Here's how the part is built. I have some questions about the finished solid (model axes, mm). Face numbers are marked on the shaded views. Give positions to 0.01 mm unless a question says otherwise; leave off trailing zeros. Loops run counter-clockwise (first coordinate to the right, second up) from the corner with the lowest first, then second, coordinate; pieces in that order, holes last. Notation, with made-up numbers: (-19, -30) - (17, -30) arc R21 cw to (17, -19) - close; hole circle Ø11 at (49.25, 32). An arc over 180 degrees is marked (long way). Use one line per item in the form item = value.
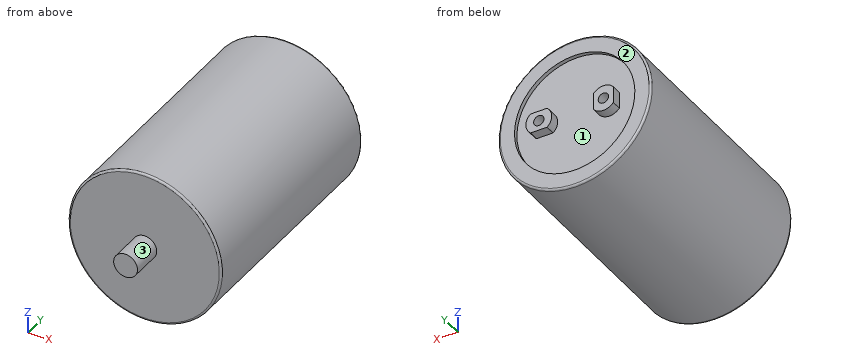
from build123d import *

# Parameters (mm, degrees)
SKETCH1_R           = 38.5
BOSS_EXTRUDE1_DEPTH = 115
SKETCH2_R           = 2.6
BOSS_EXTRUDE2_DEPTH = 5
SKETCH3_R           = 38.5
SKETCH3_R_2         = 30.3
BOSS_EXTRUDE3_DEPTH = 2
FILLET1_R           = 1
ESQUISSE1_R         = 6
BOSS_EXTRU_1_DEPTH  = 16


with BuildPart() as part:
    # Sketch1 → Boss-Extrude1 (new body)
    with BuildSketch(Plane(origin=(0, 0, 0), x_dir=(1, 0, 0), z_dir=(0, 1, 0))):
        with Locations(Location((0, 0, 0), (0, 0, 270))):
            Circle(SKETCH1_R)
    extrude(amount=BOSS_EXTRUDE1_DEPTH)

    # Sketch2 → Boss-Extrude2 (add)
    # profile 1 of 2: a face of its own
    with BuildSketch(Plane(origin=(0, 115, 0), x_dir=(1, 0, 0), z_dir=(0, 1, 0))):
        with BuildLine():
            Line((-21.25, 4.153311931), (-21.25, -4.153311931))
            ThreePointArc((-21.25, -4.153311931), (-16.25, -6.5), (-11.25, -4.153311931))
            Line((-11.25, -4.153311931), (-11.25, 4.153311931))
            ThreePointArc((-11.25, 4.153311931), (-16.25, 6.5), (-21.25, 4.153311931))
        make_face()
        with Locations(Location((-16.25, 0, 0), (0, 0, 270))):
            Circle(SKETCH2_R, mode=Mode.SUBTRACT)
    # profile 2 of 2: a face of its own
    with BuildSketch(Plane(origin=(0, 115, 0), x_dir=(1, 0, 0), z_dir=(0, 1, 0))):
        with BuildLine():
            Line((12.096688069, 5), (20.403311931, 5))
            ThreePointArc((20.403311931, 5), (22.75, 0), (20.403311931, -5))
            Line((20.403311931, -5), (12.096688069, -5))
            ThreePointArc((12.096688069, -5), (9.75, 0), (12.096688069, 5))
        make_face()
        with Locations(Location((16.25, 0, 0), (0, 0, 270))):
            Circle(SKETCH2_R, mode=Mode.SUBTRACT)
    extrude(amount=BOSS_EXTRUDE2_DEPTH)

    # Sketch3 → Boss-Extrude3 (add)
    with BuildSketch(Plane(origin=(0, 115, 0), x_dir=(1, 0, 0), z_dir=(0, 1, 0))):
        with Locations(Location((0, 0, 0), (0, 0, 270))):
            Circle(SKETCH3_R)
        with Locations(Location((0, 0, 0), (0, 0, 270))):
            Circle(SKETCH3_R_2, mode=Mode.SUBTRACT)
    extrude(amount=BOSS_EXTRUDE3_DEPTH)

    # Fillet1
    fillet1_edges = [part.edges().sort_by_distance(p)[0] for p in [
        (0, 0, -38.5),
        (0, 117, -38.5),
    ]]
    fillet(fillet1_edges, radius=FILLET1_R)

    # Esquisse1 → Boss.-Extru.1 (add)
    with BuildSketch(Plane.XZ):
        with Locations(Location((0, 0, 0), (0, 0, 90))):
            Circle(ESQUISSE1_R)
    extrude(amount=BOSS_EXTRU_1_DEPTH)


solid = part.part
(1) If I drill on probe 1 along X at (y, z) = (116.8, 0); probe 2 along X at (y, z) = (116, 0); probe 3 along Z at (x, y) = (-1, 79.5), over which ranges is the centre line in solid material (lowest first)?
Geometry says:
probe_1 = -38.1 to -30.3, -21.25 to -18.85, -13.65 to -11.25, 9.75 to 13.65, 18.85 to 22.75, 30.3 to 38.1
probe_2 = -38.5 to -30.3, -21.25 to -18.85, -13.65 to -11.25, 9.75 to 13.65, 18.85 to 22.75, 30.3 to 38.5
probe_3 = -38.49 to 38.49
(2) If we section it at C-C (y = 41.5): List the corners of the cut face in (x, z) for me.
Geometry says:
outline = circle Ø77 at (0, 0)
(3) Thinking about a two-plate mould opening in X: for the marked faces 1, 2 and 3, which applies, pulls with the +X half, pulls with the -X half, needs draft (parallel to the pull), parting line crosses it, or undercut?
Geometry says:
face_1 = undercut
face_2 = needs draft
face_3 = parting line crosses it
(4) For P1, Ø10, axis at y = 88.5, z = -26, coming from the -X side; P2, Ø1.5, axis at y = 117, z = -1.5, coming from the -X side; P3, Ø6, axis at x = 10.5, z = 22.5, coming from the -Y side, each with a flat end and sliding along its axis, tell me the tip position at first contact or that it passes through.
Geometry says:
P1 = -32.27
P2 = -38.44
P3 = 0
(5) If we section it at B-B (x = 0): List the corners of the cut face in (y, z) for me, plus the area to 3 significant figures.
Geometry says:
outline = (-16, -6) - (0, -6) - (0, -37.5) arc R1 ccw to (1, -38.5) - (116, -38.5) arc R1 ccw to (117, -37.5) - (117, -30.3) - (115, -30.3) - (115, 30.3) - (117, 30.3) - (117, 37.5) arc R1 ccw to (116, 38.5) - (1, 38.5) arc R1 ccw to (0, 37.5) - (0, 6) - (-16, 6) - close
area = 9,080 mm²
